from build123d import *

# Parameters (mm, degrees)
ESQUISSE1_R        = 15
BOSS_EXTRU_1_DEPTH = 27
ESQUISSE2_R        = 10
BOSS_EXTRU_2_DEPTH = 67
CHANFREIN1_SIZE    = 1
CONG_1_R           = 1.5


with BuildPart() as part:
    # Esquisse1 → Boss.-Extru.1 (new body)
    with BuildSketch(Plane.XY):
        Circle(ESQUISSE1_R)
    extrude(amount=BOSS_EXTRU_1_DEPTH)

    # Esquisse2 → Boss.-Extru.2 (add)
    with BuildSketch(Plane(origin=(0, 0, 0), x_dir=(-1, 0, 0), z_dir=(0, 0, -1))):
        with Locations(Location((0, 0, 0), (0, 0, 180))):  # turned: the seam where the file's is
            Circle(ESQUISSE2_R)
    extrude(amount=BOSS_EXTRU_2_DEPTH)

    # Chanfrein1
    chanfrein1_edges = [part.edges().sort_by_distance(p)[0] for p in [
        (-15, 0, 0),
        (-15, 0, 27),
        (-10, 0, -67),
    ]]
    chamfer(chanfrein1_edges, length=CHANFREIN1_SIZE)

    # Congé1
    cong_1_edges = [part.edges().sort_by_distance(p)[0] for p in [
        (-10, 0, 0),
    ]]
    fillet(cong_1_edges, radius=CONG_1_R)


solid = part.part
Geometry: final body of the model. Coordinates: model frame, mm. A direction names the side the tool comes from. Give positions to 0.01 mm unless a question says otherwise; leave off trailing zeros. Loops run counter-clockwise (first coordinate to the right, second up) from the corner with the lowest first, then second, coordinate; pieces in that order, holes last. Notation, with made-up numbers: M 85,13 L 132,13 A25 cw 132,47 Z; hole C 42.25,51 d2. An arc over 180 degrees is marked long. Put each result on its own line as item: value. Start each with the question number.
1) Cut plane A-A (y = 0). Output: boundary loops of the cut face in (x, z).
2) Cut plane D-D (z = 13). Output: boundary loops of the cut face in (x, y).
3) Ray query, line 1 along Z through (x, y) = (6, 10.5); line 2 along Y through (x, z) = (-0.5, 10.5); line 3 along Y through (x, z) = (12, 14). Return the intervals inside material, ascending.
4) Access query for faces 1 (the flat face through (0, 0, -67)), 2 (the flat face through (2, 11.5, 0)). Directions: +Z, -Z, +X, -X, +Y, -Y. A direction counts if a zero-diameter tool reaches every point of the face in a straight line with its end or side. Return the directions, or none.
5) Cut plane C-C (z = -27). Output: boundary loops of the cut face in (x, y), then the cut area to 3 significant figures.
6) Contact query for flat-ended pins moving along their axis: pin 1 (6 mm diameter, centred on y = -6, z = -46, fed in from +X); pin 2 (4 mm diameter, centred on y = -7, z = -47.5, fed in from -X); pin 3 (10 mm diameter, centred on y = 5, z = -45.5, fed in from -X). Output: stop coordinate, or through.
Verdict:
1. outline: M -15,1 L -14,0 L -11.5,0 A1.5 cw -10,-1.5 L -10,-66 L -9,-67 L 9,-67 L 10,-66 L 10,-1.5 A1.5 cw 11.5,0 L 14,0 L 15,1 L 15,26 L 14,27 L -14,27 L -15,26 Z
2. outline: C 0,0 d30
3. line 1: 0 to 27
3. line 2: -14.99 to 14.99
3. line 3: -9 to 9
4. face 1: -Z, +X, -X, +Y, -Y
4. face 2: -Z
5. outline: C 0,0 d20
5. area: 314 mm2
6. pin 1: x = 9.54
6. pin 2: x = -8.66
6. pin 3: x = -10
